Can you work these out from the model? Positions are in its coordinate system, mm. Round coordinates to 2 decimals unless told otherwise and drop trailing zeros. Loops run counter-clockwise (first coordinate to the right, second up) from the corner with the lowest first, then second, coordinate; pieces in that order, holes last. Notation, with made-up numbers: M 73,-27.5 L 82,-27.5 A13 cw 82,-15.5 Z; hole C 33.5,17.5 d11. An arc over 180 degrees is marked long. Return JSON: item names as keys, results as strings.
```python
from build123d import *

# Parameters (mm, degrees)
BOX244_W                  = 0.5
BOX244_H                  = 1
BOX244_DEPTH              = 15
BOX244_ROLL_ANGLE         = 46
BOX245_W                  = 0.5
BOX245_H                  = 1
BOX245_DEPTH              = 15
BOX245_ROLL_ANGLE         = -46
BOX243_W                  = 0.5
BOX243_H                  = 1
BOX243_DEPTH              = 11
FUSION024_PLACEMENT_ANGLE = 46.5


with BuildPart() as cubo244:
    # Box244 → Box244 (new body)
    with BuildSketch(Plane.XY):
        with Locations((0.25, 0.5)):
            Rectangle(BOX244_W, BOX244_H)
    extrude(amount=BOX244_DEPTH)


with BuildPart() as cubo244_1:
    # Box244 roll: moved
    add(cubo244.part.rotate(Axis((0, 0, 0), (1, 0, 0)), BOX244_ROLL_ANGLE))


with BuildPart() as cubo244_2:
    # Box244 placement: moved
    add(cubo244_1.part.moved(Location((0, 11, 0.5))))


with BuildPart() as cubo245:
    # Box245 → Box245 (new body)
    with BuildSketch(Plane.XY):
        with Locations((0.25, 0.5)):
            Rectangle(BOX245_W, BOX245_H)
    extrude(amount=BOX245_DEPTH)


with BuildPart() as cubo245_1:
    # Box245 roll: moved
    add(cubo245.part.rotate(Axis((0, 0, 0), (1, 0, 0)), BOX245_ROLL_ANGLE))


with BuildPart() as cubo245_2:
    # Box245 placement: moved
    add(cubo245_1.part.moved(Location((0, 0.4, 1.1))))


with BuildPart() as fusion024:
    # Box243 → Box243 (new body)
    with BuildSketch(Plane.XY.offset(0.5)):
        with Locations((0.25, 0.5)):
            Rectangle(BOX243_W, BOX243_H)
    extrude(amount=BOX243_DEPTH)

    # Fusion024: union Cubo244, Cubo245
    add(cubo244_2.part)
    add(cubo245_2.part)


with BuildPart() as fusion024_1:
    # Fusion024 placement: moved
    add(fusion024.part.moved(Location((-163.4, 167.7, 0))).rotate(Axis((-163.4, 167.7, 0), (0, 0, -1)), FUSION024_PLACEMENT_ANGLE))


solid = fusion024_1.part
```
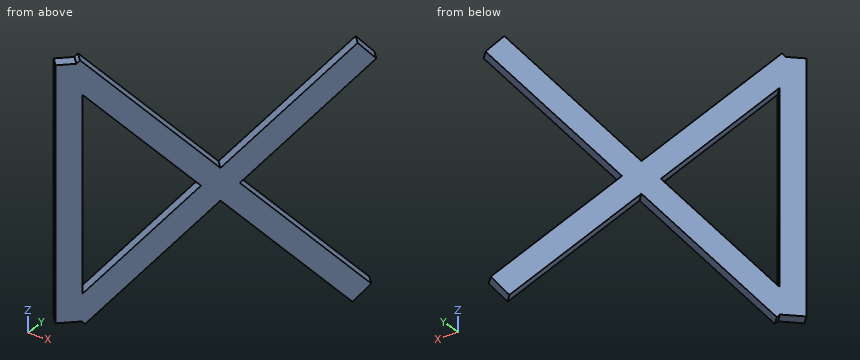
Q1. If I drill on line 1 along X through (y, z) = (168.25, 4); line 2 along Y through (x, z) = (-156.75, 8.75); line 3 along X through (y, z) = (168, 4.25), over which ranges is the centre line in solid material (lowest first)?
Results:
{"line 1": "x = -162.82 to -162.54", "line 2": "y = 173.32 to 174.01", "line 3": "x = -163.08 to -162.36"}
Q2. Suppose I cut it at B-B, the plane z = 2. Please give me the cut outline in (x, y).
Results:
{"outline": "M -163.4,167.7 L -163.06,167.34 L -162.33,168.03 L -162.67,168.39 Z; M -162.43,168.62 L -162.09,168.25 L -161.05,169.25 L -161.39,169.61 Z; M -156.55,174.2 L -156.2,173.84 L -155.16,174.83 L -155.5,175.19 Z"}
Q3. Suppose I cut it at C-C, the plane x = -157.5. Please give me the cut outline in (y, z), plus the area to 3 significant figures.
Results:
{"outline": "M 172.61,3.73 L 173.3,3.27 L 173.3,4.66 L 172.61,5.12 Z; M 172.61,6.72 L 173.3,7.18 L 173.3,8.57 L 172.61,8.11 Z", "area": "1.92 mm2"}
Q4. I'm going to push flat-ended pins straight in: pin 1 Ø4 at (x, z) = (-159.5, 8) entering from +Y; pin 2 Ø4 at (y, z) = (171.5, 2.5) entering from +X; pin 3 Ø2 at (y, z) = (171.5, 6.5) entering from +X. Where does each tip first touch, or does it pass through?
Results:
{"pin 1": "stops at y = 173.3", "pin 2": "stops at x = -156.56", "pin 3": "stops at x = -157.62"}
Q5. Suppose I cut it at A-A, the plane z = 5.5. Please give me the cut outline in (x, y), plus the area to 3 significant figures.
Results:
{"outline": "M -163.4,167.7 L -163.06,167.34 L -162.33,168.03 L -162.67,168.39 Z; M -159.8,171.11 L -159.46,170.75 L -157.79,172.34 L -158.13,172.7 Z", "area": "1.65 mm2"}
